Source: CAD feature listing. Evaluate the final solid. Frame: model axes, mm. A direction names the side the tool comes from. Give positions to 0.01 mm unless a question says otherwise; leave off trailing zeros. Order: outer loops, then holes, each group sorted by start corner. A loop starts at its lowest first (then second) coordinate and runs counter-clockwise, first axis right, second up.
from build123d import *

# Parameters (mm, degrees)
SKETCH1_R           = 11.049
BOSS_EXTRUDE1_DEPTH = 63.5
SKETCH2_W           = 177.8
SKETCH2_H           = 31.75
CUT_EXTRUDE1_DEPTH  = 138.407720282


with BuildPart() as part:
    # Sketch1 → Boss-Extrude1 (new body)
    with BuildSketch(Plane(origin=(0, 0, 0), x_dir=(1, 0, 0), z_dir=(0, 1, 0))):
        with BuildLine():
            Line((-87.191795428, 59.02921057), (87.191795428, 59.02921057))
            ThreePointArc((87.191795428, 59.02921057), (118.872, 49.50421057), (87.191795428, 39.97921057))
            Line((87.191795428, 39.97921057), (-87.191795428, 39.97921057))
            ThreePointArc((-87.191795428, 39.97921057), (-118.872, 49.50421057), (-87.191795428, 59.02921057))
        make_face()
        with Locations(Location((101.6, 49.50421057, 0), (0, 0, 270))):
            Circle(SKETCH1_R, mode=Mode.SUBTRACT)
        with Locations(Location((-101.6, 49.50421057, 0), (0, 0, 270))):
            Circle(SKETCH1_R, mode=Mode.SUBTRACT)
    extrude(amount=BOSS_EXTRUDE1_DEPTH)

    # Sketch2 → Cut-Extrude1 (cut, through all)
    with BuildSketch(Plane.XY.offset(-39.97921057)):
        with Locations((0, 31.75)):
            Rectangle(SKETCH2_W, SKETCH2_H)
    extrude(amount=-CUT_EXTRUDE1_DEPTH, mode=Mode.SUBTRACT)


solid = part.part
(1) Section B-B, the plane z = -56.5. Return loops of the section in (x, y) (3 decimals).
(2) Access query for faces 4 (the cylindrical face through (-94.133, 31.306, -57.648)), 5 (the flat face through (1, 8, -39.979)), 6 (the flat face through (88.9, 32, -50)), 7 (the flat face through (-1, 8, -59.029)). Directions: +Z, -Z, +X, -X, +Y, -Y. A direction counts if a zero-diameter tool reaches every point of the face in a straight line with its end or side. Return the directions, or none.
(3) Section A-A, the plane y = 45. Return loops of the section in (x, z), plus the area to 3 significant figures.
(4) Line query: line 1 along X through (y, z) = (20, -50); line 2 along Y through (x, z) = (46.5, -45.5) (3 decimals); line 3 along X through (y, z) = (4, -42). Output: solid intervals per line, ascending.
(5) Section C-C, the plane x = -101.6. Return loops of the section in (y, z).
(6) Draft query along Z for faces 1 (the cylindrical face through (118.86, 31.31, -50.12)), 2 (the cylindrical face through (109.067, 31.306, -57.648)), 3 (the flat face through (1, 55, -39.979)). Return one class per face: +Z half, -Z half, draft (parallel to the pull), parting line (faces both ways), or undercut.
(7) Section D-D, the plane x = 39. Return loops of the section in (y, z) (3 decimals), plus the area to 3 significant figures.
(8) Pin query (flat end, axial travel): pin 1 Ø17.5 at (x, y) = (-40.5, 58.5) entering from -Z; pin 2 Ø17.5 at (x, y) = (4.5, 12) entering from +Z; pin 3 Ø0.5 at (x, y) = (-87.5, 35.5) entering from -Z. Return the tip coordinate at first contact, or that it passes through.
Checks:
1. outline: (-117.392, 0) - (-110.152, 0) - (-110.152, 63.5) - (-117.392, 63.5) - close; (-93.048, 0) - (93.048, 0) - (93.048, 63.5) - (-93.048, 63.5) - close; (110.152, 0) - (117.392, 0) - (117.392, 63.5) - (110.152, 63.5) - close; hole (-88.9, 15.875) - (88.9, 15.875) - (88.9, 47.625) - (-88.9, 47.625) - close
2. face 4: +Y, -Y
2. face 5: +Z, +Y, -Y
2. face 6: -Z
2. face 7: -Z, +Y, -Y
3. outline: (-88.9, -61.21) - (-88.9, -39.98) - (-87.19, -39.98) arc R17.27 ccw (long way) to start; (87.19, -39.98) - (88.9, -39.98) - (88.9, -61.21) arc R17.27 ccw (long way) to start; hole circle Ø22.1 at (-101.6, -49.5); hole circle Ø22.1 at (101.6, -49.5)
3. area: 964 mm2
4. line 1: x = -118.86 to -112.64, -90.56 to -88.9, 88.9 to 90.56, 112.64 to 118.86
4. line 2: y = 0 to 15.875, 47.625 to 63.5
4. line 3: x = -117.16 to -109.71, -93.49 to 93.49, 109.71 to 117.16
5. outline: (0, -66.78) - (63.5, -66.78) - (63.5, -60.55) - (0, -60.55) - close; (0, -38.46) - (63.5, -38.46) - (63.5, -32.23) - (0, -32.23) - close
6. face 1: parting line
6. face 2: undercut
6. face 3: +Z half
7. outline: (0, -59.029) - (15.875, -59.029) - (15.875, -39.979) - (0, -39.979) - close; (47.625, -59.029) - (63.5, -59.029) - (63.5, -39.979) - (47.625, -39.979) - close
7. area: 605 mm2
8. pin 1: stops at z = -59.03
8. pin 2: stops at z = -39.98
8. pin 3: stops at z = -39.98
